Part print with two shaded views. Sizes in mm from the minimum x, y, z corner. Coordinates: 2 decimals unless noted, no trailing zeros. Order: outer loops, then holes, each group sorted by start corner. A loop starts at its lowest first (then second) coordinate and runs counter-clockwise, first axis right, second up. Notation, with made-up numbers: (-32, 57) - (-28, 57) arc R25 ccw to (-28, 91) - close; hole circle Ø9 at (54, 12). An arc over 180 degrees is marked (long way). Write each question's results on one line, items separated by ' | '. Start each with the question number.
Q1. Wall check: probe 1 along X at (y, z) = (1.2, 50); probe 2 along X at (y, z) = (2.8, 50); probe 3 along Y at (x, z) = (96, 35). Give the ranges that are in metal, low to high.
Q2. Band-saw the part on A-A, the plane z = 50. Write the cut outline in (x, y).
Q3. Pin check, flat tips, straight feed: P1, Ø2, axis at x = 36, y = 0.5, coming from the -Z side; P2, Ø1, axis at x = 62, y = 1, coming from the +Z side. Stop position of each tip, or through.
Q4. Band-saw the part on C-C, the plane y = 1.4. Write the cut outline in (x, z), then the cut area to 3 significant figures.
Q5. Band-saw the part on D-D, the plane x = 6. Write the cut outline in (y, z).
Q6. Band-saw the part on B-B, the plane x = 30. Write the cut outline in (y, z).
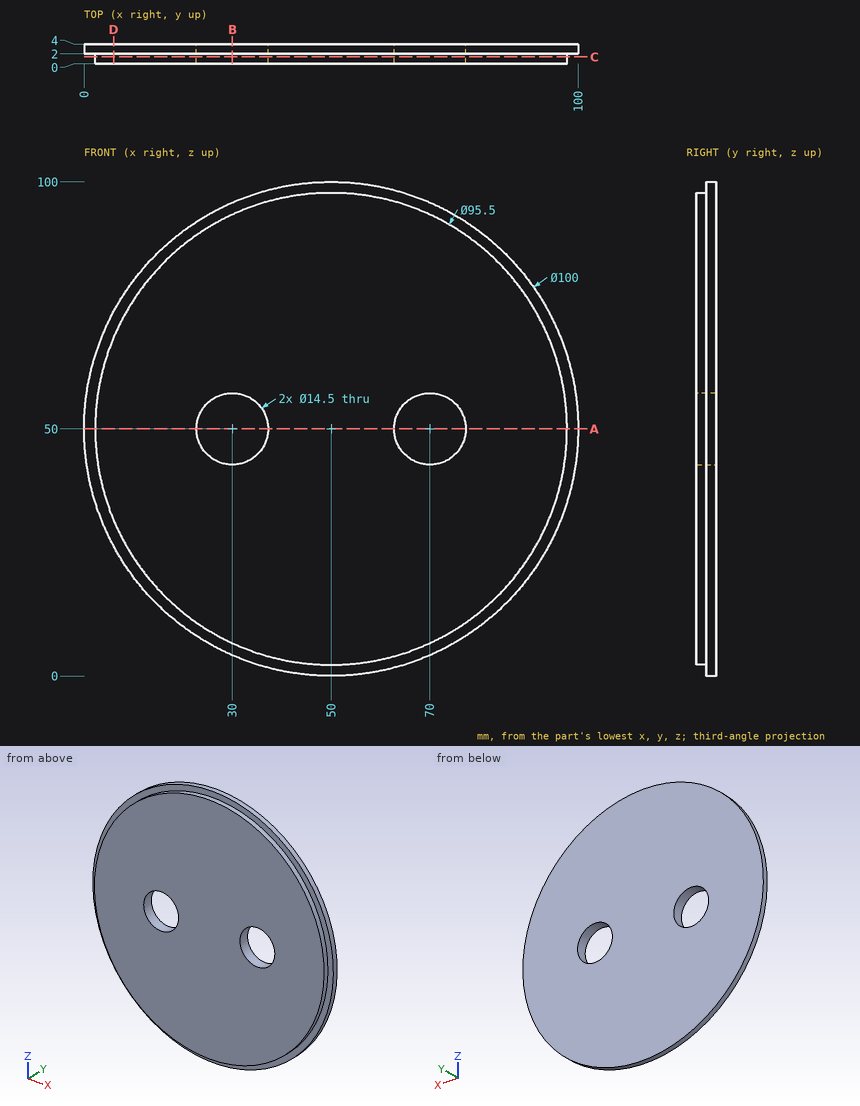
Results below:
1) probe 1: x = 2.25 to 22.75, 37.25 to 62.75, 77.25 to 97.75 | probe 2: x = 0 to 22.75, 37.25 to 62.75, 77.25 to 100 | probe 3: y = 2 to 4
2) outline: (0, 2) - (2.25, 2) - (2.25, 0) - (22.75, 0) - (22.75, 4) - (0, 4) - close; (37.25, 0) - (62.75, 0) - (62.75, 4) - (37.25, 4) - close; (77.25, 0) - (97.75, 0) - (97.75, 2) - (100, 2) - (100, 4) - (77.25, 4) - close
3) P1: stops at z = 4.05 | P2: stops at z = 96.34
4) outline: circle Ø95.5 at (50, 50); hole circle Ø14.5 at (30, 50); hole circle Ø14.5 at (70, 50) | area: 6,830 mm²
5) outline: (0, 31.45) - (2, 31.45) - (2, 26.25) - (4, 26.25) - (4, 73.75) - (2, 73.75) - (2, 68.55) - (0, 68.55) - close
6) outline: (0, 6.64) - (2, 6.64) - (2, 4.17) - (4, 4.17) - (4, 42.75) - (0, 42.75) - close; (0, 57.25) - (4, 57.25) - (4, 95.83) - (2, 95.83) - (2, 93.36) - (0, 93.36) - close
